```python
from build123d import *

# Parameters (mm, degrees)
SKETCH1_R         = 150
DISC_DEPTH        = 4
SKETCH2_R         = 20
HUB_DEPTH         = 20
SKETCH3_R         = 4
BORE_DEPTH        = 24
SKETCH4_W         = 71.782300335
SKETCH4_H         = 3
BLADE_SLOTS_DEPTH = 3
SKETCH5_R         = 1.25
CLAMP_SCREW_DEPTH = 17


with BuildPart() as part:
    # Sketch1 → Disc (new body)
    with BuildSketch(Plane.XY):
        Circle(SKETCH1_R)
    extrude(amount=DISC_DEPTH)

    # Sketch2 → Hub (add)
    with BuildSketch(Plane.XY.offset(4)):
        Circle(SKETCH2_R)
    extrude(amount=HUB_DEPTH)

    # Sketch3 → Bore (cut)
    with BuildSketch(Plane.XY):
        Circle(SKETCH3_R)
    extrude(amount=BORE_DEPTH, mode=Mode.SUBTRACT)

    # Sketch4 → Blade_slots (cut)
    with BuildSketch(Plane.XY):
        with Locations((63.2155163, -96.418141453)):
            Rectangle(SKETCH4_W, SKETCH4_H)
        Polygon((83.872246927, -57.445884148), (138.860679213, -11.305110898), (136.932316384, -9.006977568), (81.943884098, -55.147750818), align=None)
        Polygon((101.175371248, 9.90594079), (113.64023689, 80.597706689), (110.685813631, 81.118651222), (98.220947989, 10.426885323), align=None)
        Polygon((71.137414923, 72.62266594), (35.246264756, 134.787961572), (32.648188544, 133.287961572), (68.539338712, 71.12266594), align=None)
        Polygon((7.813471551, 101.358438585), (-59.639826377, 125.909431234), (-60.665886807, 123.090353372), (6.787411121, 98.539360723), align=None)
        Polygon((-59.166481997, 82.667471343), (-126.619779924, 58.116478695), (-125.593719494, 55.297400832), (-58.140421567, 79.848393481), align=None)
        Polygon((-98.461781056, 25.295475513), (-134.352931224, -36.869820119), (-131.754855012, -38.369820119), (-95.863704845, 23.795475513), align=None)
        Polygon((-91.685718479, -43.912554438), (-79.220852837, -114.604320337), (-76.266429578, -114.083375804), (-88.73129522, -43.391609905), align=None)
        Polygon((-42.008889252, -92.573412133), (12.979543034, -138.714185383), (14.907905863, -136.416052054), (-40.080526423, -90.275278804), align=None)
    extrude(amount=BLADE_SLOTS_DEPTH, mode=Mode.SUBTRACT)

    # Sketch5 → Clamp_screw (cut)
    with BuildSketch(Plane(origin=(3.5, 0, 0), x_dir=(0, 0, -1), z_dir=(1, 0, 0))):
        with Locations(Location((-14, 0, 0), (0, 0, 180))):
            Circle(SKETCH5_R)
    extrude(amount=CLAMP_SCREW_DEPTH, mode=Mode.SUBTRACT)


solid = part.part
```
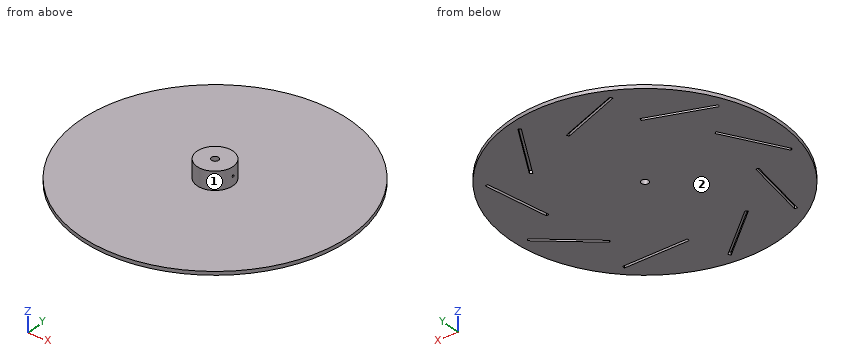
For this review, take the finished solid that the model builds, in its own axes (mm). Face numbers are marked on the shaded views. A direction names the side the tool comes from. Coordinates: 2 decimals unless noted, no trailing zeros. Order: outer loops, then holes, each group sorted by start corner. A loop starts at its lowest first (then second) coordinate and runs counter-clockwise, first axis right, second up. Notation, with made-up numbers: (-15, 38) - (28, 38) arc R21 cw to (28, 67) - close; hole circle Ø7 at (27.5, 62). An arc over 180 degrees is marked (long way). Answer as a JSON object with one key per item and string values. Group by question number.
1. For the marked faces 1 and 2, list the 3-axis set-ups (+Z, -Z, +X, -X, +Y, -Y) from which the entire face can be reached by the end or side of a thin tool; tool diameter is ignored.
2. We need section A-A on z = 20.25. State the section outline as (x, y) points, then the cut area to 3 significant figures.
3. Clearance check with flat-ended pins moving along their axes: P1, Ø3, axis at y = 1, z = 16, coming from the +X side; P2, Ø5, axis at x = -8, y = 40.5, coming from the +Z side; P3, Ø1.5, axis at x = 46.5, z = 1.5, coming from the -Y side; P4, Ø2, axis at y = -79, z = 6, coming from the -X side. State where each tip first meets the part, or that it passes through.
4. For probe 1 along Y at (x, z) = (0, 16.5); probe 2 along Y at (x, z) = (40.5, 2.75); probe 3 along Z at (x, y) = (-38, -102), list the stretches that pass through material, from the lowest coordinate up.
5. We need section B-B on x = 0. State the section outline as (y, z) points.
6. We need section C-C on x = -114. State the section outline as (y, z) points.
Final values:
{
 "1": {"face 1": "+Z", "face 2": "-Z, +X, -X, +Y, -Y"},
 "2": {"outline": "circle Ø40 at (0, 0); hole circle Ø8 at (0, 0)", "area": "1,210 mm²"},
 "3": {"P1": "x = 20", "P2": "z = 4", "P3": "y = -142.85", "P4": "through"},
 "4": {"probe 1": "-20 to -4, 4 to 20", "probe 2": "-144.43 to -97.92, -94.92 to 119.69, 125.69 to 144.43", "probe 3": "0 to 4"},
 "5": {"outline": "(-150, 0) - (-127.82, 0) - (-127.82, 3) - (-123.91, 3) - (-123.91, 0) - (-4, 0) - (-4, 24) - (-20, 24) - (-20, 4) - (-150, 4) - close; (4, 0) - (101.01, 0) - (101.01, 3) - (104.2, 3) - (104.2, 0) - (150, 0) - (150, 4) - (20, 4) - (20, 24) - (4, 24) - close"},
 "6": {"outline": "(-97.49, 0) - (-7.62, 0) - (-7.62, 3) - (-1.62, 3) - (-1.62, 0) - (59.52, 0) - (59.52, 3) - (62.71, 3) - (62.71, 0) - (97.49, 0) - (97.49, 4) - (-97.49, 4) - close"}
}
